```python
from build123d import *

# Parameters (mm, degrees)
SKETCH_1_R             = 4
EXTRUDE_1_DEPTH        = 7.15
SKETCH_2_W             = 1
SKETCH_2_H             = 4
CHAMFER_1_SIZE         = 0.5
HOLE_WIZARD_M5_1_D     = 4.2
HOLE_WIZARD_M5_1_DEPTH = 17.4
HOLE_WIZARD_M5_1_TIP   = 1.2618073


with BuildPart() as part:
    # 草图1 → 凸台-拉伸1 (new, symmetric)
    with BuildSketch(Plane(origin=(0, 0, 0), x_dir=(1, 0, 0), z_dir=(0, 1, 0))):
        with Locations(Location((0, 0, 0), (0, 0, 270))):
            Circle(SKETCH_1_R)
    extrude(amount=EXTRUDE_1_DEPTH, both=True)

    # 草图2 → 旋转1 (revolve)
    with BuildSketch(Plane.XY, mode=Mode.PRIVATE) as revolve_1_sk:
        with Locations((4.5, -5.15)):
            Rectangle(SKETCH_2_W, SKETCH_2_H)
    revolve(revolve_1_sk.sketch.rotate(Axis((0, 7.15, 0), (0, -1, 0)), 270), axis=Axis((0, 7.15, 0), (0, -1, 0)))

    # 倒角1
    chamfer_1_edges = [part.edges().sort_by_distance(p)[0] for p in [
        (0, 7.15, -4),
    ]]
    chamfer(chamfer_1_edges, length=CHAMFER_1_SIZE)

    # M5 螺纹孔1
    with Locations(Plane(origin=(0, -7.15, 0), x_dir=(-1, 0, 0), z_dir=(0, -1, 0))):
        with Locations((0, 0)):
            Hole(HOLE_WIZARD_M5_1_D / 2, depth=HOLE_WIZARD_M5_1_DEPTH)
            with Locations((0, 0, -(HOLE_WIZARD_M5_1_DEPTH + HOLE_WIZARD_M5_1_TIP / 2))):  # 118° drill point
                Cone(0, HOLE_WIZARD_M5_1_D / 2, HOLE_WIZARD_M5_1_TIP, mode=Mode.SUBTRACT)


solid = part.part
```
Build history of the part. All positions in model axes, mm. Round coordinates to 2 decimals unless told otherwise and drop trailing zeros. Loops run counter-clockwise (first coordinate to the right, second up) from the corner with the lowest first, then second, coordinate; pieces in that order, holes last.
Item 1: Two-plate mould, pull along Z, no slides. Class faces 1 (the face through (-2.2, -7.15, 1)), 2 (the face through (2.003, 0.1, -0.631)), 3 (the face through (-3.905, 1.819, -0.867)): released by +Z, released by -Z, zero draft, split by the parting line, or undercut.
Item 2: Saw through at B-B (z = 0). List the corners of the cut face in (x, y), then the cut area to 3 significant figures.
Item 3: Drill centre lines: line 1 along Z through (x, y) = (0, 3.5); line 2 along X through (y, z) = (3.75, 0.75); line 3 along Y through (x, z) = (4, 1.5). Where is each one in solid material? Low to high.
Item 4: Saw through at C-C (y = -5.25). List the corners of the cut face in (x, z), then the cut area to 3 significant figures.
Item 5: Pin check, flat tips, straight feed: P1, Ø1, axis at x = -3.5, y = -0.5, coming from the -Z side; P2, Ø2, axis at y = 5.5, z = 3, coming from the +X side; P3, Ø4, axis at y = 1.5, z = 4, coming from the -X side. Stop position of each tip, or through.
Item 6: Saw through at A-A (x = 0). List the corners of the cut face in (y, z).
Item 7: Saw through at D-D (y = 4.5). List the corners of the cut face in (x, z), then the cut area to 3 significant figures.
Worked answers:
1. face 1: zero draft
1. face 2: undercut
1. face 3: split by the parting line
2. outline: (-5, -7.15) - (-2.1, -7.15) - (-2.1, 7.15) - (-3.5, 7.15) - (-4, 6.65) - (-4, -3.15) - (-5, -3.15) - close; (2.1, -7.15) - (5, -7.15) - (5, -3.15) - (4, -3.15) - (4, 6.65) - (3.5, 7.15) - (2.1, 7.15) - close
2. area: 62.1 mm2
3. line 1: z = -4 to -2.1, 2.1 to 4
3. line 2: x = -3.93 to -1.96, 1.96 to 3.93
3. line 3: y = -7.15 to -3.15
4. outline: circle Ø10 at (0, 0); hole circle Ø4.2 at (0, 0)
4. area: 64.7 mm2
5. P1: stops at z = -2.65
5. P2: stops at x = 3.46
5. P3: stops at x = -3.46
6. outline: (-7.15, -5) - (-3.15, -5) - (-3.15, -4) - (6.65, -4) - (7.15, -3.5) - (7.15, -2.1) - (-7.15, -2.1) - close; (-7.15, 2.1) - (7.15, 2.1) - (7.15, 3.5) - (6.65, 4) - (-3.15, 4) - (-3.15, 5) - (-7.15, 5) - close
7. outline: circle Ø8 at (0, 0); hole circle Ø4.2 at (0, 0)
7. area: 36.4 mm2
